Source: three-view drawing plus pictorial views. Frame: mm from the lowest corner of the part. Coordinates: 2 decimals unless noted, no trailing zeros. Loops run counter-clockwise (first coordinate to the right, second up) from the corner with the lowest first, then second, coordinate; pieces in that order, holes last. Notation, with made-up numbers: (52.5, 0) - (105.5, 0) arc R29 cw to (105.5, 30) - close; hole circle Ø9 at (28.5, 3.5). An arc over 180 degrees is marked (long way). Answer as CSV lines item,"result". Start each with the question number.
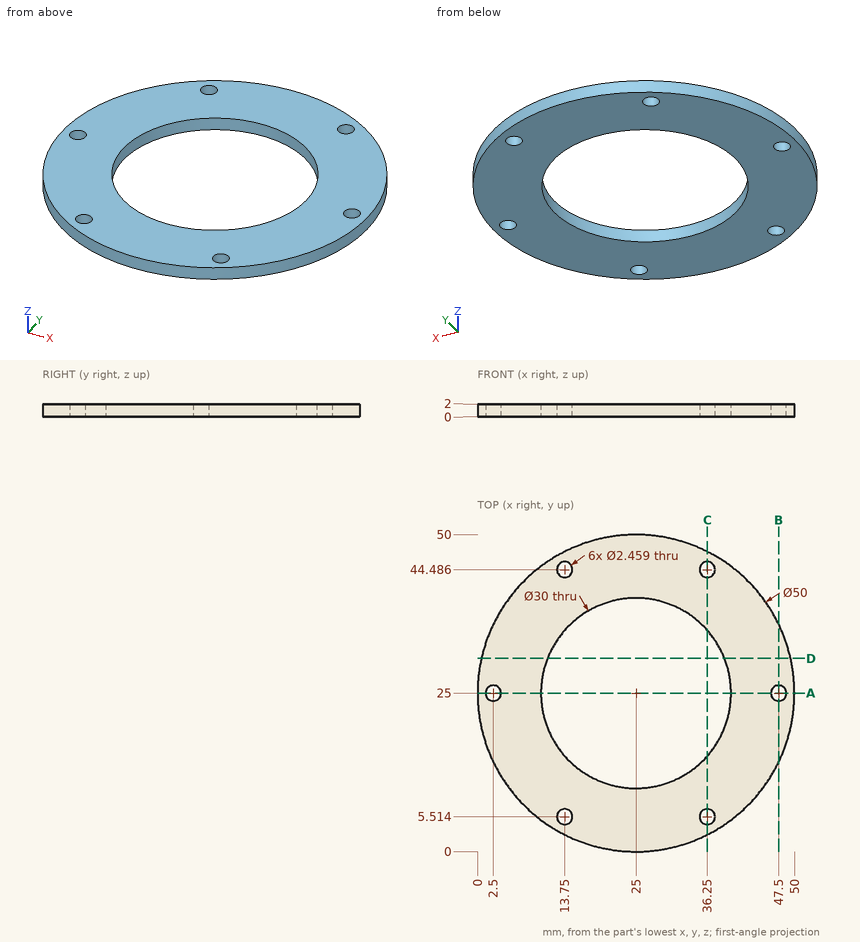
Item 1: Material intervals for probe 1 along X at (y, z) = (44, 1.4); probe 2 along X at (y, z) = (24, 1.5) (1 decimal); probe 3 along X at (y, z) = (16, 0.4) (1 decimal), sorted ascending.
Item 2: Section query C-C, the plane x = 36.25. Output: boundary loops of the cut face in (y, z) (1 decimal).
Item 3: Section query D-D, the plane y = 30.5. Output: boundary loops of the cut face in (x, z) (1 decimal).
Item 4: Contact query for a flat-ended pin moving along its axis: P1, Ø3, axis at x = 13.75, y = 44.49, coming from the +Z side. Output: stop coordinate, or through.
Item 5: Section query A-A, the plane y = 25. Output: boundary loops of the cut face in (x, z).
Item 6: Section query B-B, the plane x = 47.5. Output: boundary loops of the cut face in (y, z).
Response values:
1,probe 1,"x = 8.75 to 12.62, 14.88 to 35.12, 37.38 to 41.25"
1,probe 2,"x = 0 to 1.8, 3.2 to 10, 40 to 46.8, 48.2 to 50"
1,probe 3,"x = 1.7 to 13, 37 to 48.3"
2,outline,"(2.7, 0) - (4.3, 0) - (4.3, 2) - (2.7, 2) - close; (6.7, 0) - (15.1, 0) - (15.1, 2) - (6.7, 2) - close; (34.9, 0) - (43.3, 0) - (43.3, 2) - (34.9, 2) - close; (45.7, 0) - (47.3, 0) - (47.3, 2) - (45.7, 2) - close"
3,outline,"(0.6, 0) - (11, 0) - (11, 2) - (0.6, 2) - close; (39, 0) - (49.4, 0) - (49.4, 2) - (39, 2) - close"
4,P1,"stops at z = 2"
5,outline,"(0, 0) - (1.27, 0) - (1.27, 2) - (0, 2) - close; (3.73, 0) - (10, 0) - (10, 2) - (3.73, 2) - close; (40, 0) - (46.27, 0) - (46.27, 2) - (40, 2) - close; (48.73, 0) - (50, 0) - (50, 2) - (48.73, 2) - close"
6,outline,"(14.1, 0) - (23.77, 0) - (23.77, 2) - (14.1, 2) - close; (26.23, 0) - (35.9, 0) - (35.9, 2) - (26.23, 2) - close"
